```python
from build123d import *

# Parameters (mm, degrees)
SKETCH1_W                = 180
SKETCH1_H                = 80
BOSS_EXTRUDE1_DEPTH      = 5
BOSS_EXTRUDE2_DEPTH      = 1
BOSS_EXTRUDE2_DEPTH_BACK = 10
SKETCH1_4_W              = 180
SKETCH1_4_H              = 5
CUT_EXTRUDE3_REACH       = 195.318
SKETCH2_R                = 1.4


with BuildPart() as part:
    # Sketch1 → Boss-Extrude1 (new body)
    with BuildSketch(Plane.XY):
        with Locations((90, 40)):
            Rectangle(SKETCH1_W, SKETCH1_H)
    extrude(amount=BOSS_EXTRUDE1_DEPTH)

    # Sketch1_4 → Boss-Extrude2 (add, two sides: drawn at the far end of the back side and taken through both)
    with BuildSketch(Plane.XY.offset(-BOSS_EXTRUDE2_DEPTH_BACK)):
        with Locations((90, 7.7)):
            Rectangle(SKETCH1_4_W, SKETCH1_4_H)
    extrude(amount=BOSS_EXTRUDE2_DEPTH + BOSS_EXTRUDE2_DEPTH_BACK)

    # Sketch2 → Cut-Extrude3 (cut, up to next)
    with BuildSketch(Plane(origin=(0, 10.2, 0), x_dir=(1, 0, 0), z_dir=(0, 1, 0)), mode=Mode.PRIVATE) as cut_extrude3_sk1:
        with Locations(Location((15, 5, 0), (0, 0, 270))):
            Circle(SKETCH2_R)
    cut_extrude3_tool1 = extrude(cut_extrude3_sk1.sketch, amount=-CUT_EXTRUDE3_REACH, mode=Mode.PRIVATE) & part.part
    # Sketch2 → Cut-Extrude3 (cut, up to next)
    with BuildSketch(Plane(origin=(0, 10.2, 0), x_dir=(1, 0, 0), z_dir=(0, 1, 0)), mode=Mode.PRIVATE) as cut_extrude3_sk2:
        with Locations(Location((90, 5, 0), (0, 0, 270))):
            Circle(SKETCH2_R)
    cut_extrude3_tool2 = extrude(cut_extrude3_sk2.sketch, amount=-CUT_EXTRUDE3_REACH, mode=Mode.PRIVATE) & part.part
    # Sketch2 → Cut-Extrude3 (cut, up to next)
    with BuildSketch(Plane(origin=(0, 10.2, 0), x_dir=(1, 0, 0), z_dir=(0, 1, 0)), mode=Mode.PRIVATE) as cut_extrude3_sk3:
        with Locations(Location((165, 5, 0), (0, 0, 270))):
            Circle(SKETCH2_R)
    cut_extrude3_tool3 = extrude(cut_extrude3_sk3.sketch, amount=-CUT_EXTRUDE3_REACH, mode=Mode.PRIVATE) & part.part
    add(cut_extrude3_tool1.solids().sort_by_distance((15, 10.2, -5))[0], mode=Mode.SUBTRACT)
    add(cut_extrude3_tool2.solids().sort_by_distance((90, 10.2, -5))[0], mode=Mode.SUBTRACT)
    add(cut_extrude3_tool3.solids().sort_by_distance((165, 10.2, -5))[0], mode=Mode.SUBTRACT)


solid = part.part
```
Here's how the part is built. I have some questions about the finished solid (model axes, mm). A direction names the side the tool comes from. Give positions to 0.01 mm unless a question says otherwise; leave off trailing zeros. Write each loop counter-clockwise with the first axis right and the second up, starting at its lowest first coordinate (ties: lowest second). Pieces come first, ordered by that corner, then holes.
(1) If I drill on L1, parallel to X at y = 8.6, z = -5; L2, parallel to Z at x = 90, y = 6.7; L3, parallel to Y at x = 132, z = -0.5, over which ranges is the centre line in solid material (lowest first)?
Output values:
L1: x = 0 to 13.6, 16.4 to 88.6, 91.4 to 163.6, 166.4 to 180
L2: z = -10 to -6.4, -3.6 to 5
L3: y = 5.2 to 10.2
(2) On a 3-axis mill with a long thin cutter (end or side, diameter ignored), from which of +Z, -Z, +X, -X, +Y, -Y can I reach the whole of each face in a straight line? I mean faces 1 (the face through (88.7, 5.2, -4)), 2 (the face through (89, 46, 0)), 3 (the face through (89, 8, -10)). Say none if no direction works.
Output values:
face 1: -Z, +X, -X, -Y
face 2: -Z, +X, -X, +Y
face 3: -Z, +X, -X, +Y, -Y
(3) Will these pins go through, and if not, where does the flat tip stop? pin 1 (4.5 mm diameter, centred on x = 90, z = -5, fed in from -Y); pin 2 (3.5 mm diameter, centred on x = 165, z = -5, fed in from +Y); pin 3 (12 mm diameter, centred on x = 97, y = 22.5, fed in from -Z); pin 4 (6 mm diameter, centred on y = 44, z = 0, fed in from -X).
Output values:
pin 1: stops at y = 5.2
pin 2: stops at y = 10.2
pin 3: stops at z = 0
pin 4: stops at x = 0
(4) Imagine slicing it at B-B, the plane y = 59. Write out the boundary of the cut face in (x, z).
Output values:
outline: (0, 0) - (180, 0) - (180, 5) - (0, 5) - close
(5) Imagine slicing it at A-A, the plane x = 115. Write out the boundary of the cut face in (y, z), and give its area (3 significant figures).
Output values:
outline: (0, 0) - (5.2, 0) - (5.2, -10) - (10.2, -10) - (10.2, 0) - (80, 0) - (80, 5) - (0, 5) - close
area: 450 mm2
